```python
from build123d import *

# Parameters (mm, degrees)
BOSS_EXTRUDE1_DEPTH = 50.8
SKETCH4_R           = 2.667
CUT_EXTRUDE1_DEPTH  = 117.743329574
SKETCH5_W           = 88.9
SKETCH5_H           = 38.1
CUT_EXTRUDE2_DEPTH  = 20.32
SKETCH6_W           = 88.9
SKETCH6_H           = 38.1
CUT_EXTRUDE3_DEPTH  = 20.32
SKETCH7_R           = 3.175
CUT_EXTRUDE4_DEPTH  = 117.743329574


with BuildPart() as part:
    # Sketch3 → Boss-Extrude1 (new body)
    with BuildSketch(Plane.XY):
        Polygon((0, 6.35), (88.9, 44.45), (95.25, 44.45), (95.25, 0), (0, 0), align=None)
        Polygon((16.120053074, 6.35), (88.9, 6.35), (88.9, 37.541405825), align=None, mode=Mode.SUBTRACT)
    extrude(amount=BOSS_EXTRUDE1_DEPTH)

    # Sketch4 → Cut-Extrude1 (cut, through all)
    with BuildSketch(Plane.XZ):
        with Locations(Location((6.35, 38.1, 0), (0, 0, 270))):
            Circle(SKETCH4_R)
        with Locations(Location((6.35, 12.7, 0), (0, 0, 270))):
            Circle(SKETCH4_R)
        with Locations(Location((69.85, 12.7, 0), (0, 0, 270))):
            Circle(SKETCH4_R)
        with Locations(Location((69.85, 38.1, 0), (0, 0, 270))):
            Circle(SKETCH4_R)
    extrude(amount=-CUT_EXTRUDE1_DEPTH, mode=Mode.SUBTRACT)

    # Sketch5 → Cut-Extrude2 (cut)
    with BuildSketch(Plane.XY.offset(50.8)):
        with Locations((44.45, 25.4)):
            Rectangle(SKETCH5_W, SKETCH5_H)
    extrude(amount=-CUT_EXTRUDE2_DEPTH, mode=Mode.SUBTRACT)

    # Sketch6 → Cut-Extrude3 (cut)
    with BuildSketch(Plane(origin=(0, 0, 0), x_dir=(-1, 0, 0), z_dir=(0, 0, -1))):
        with Locations((-44.45, 25.4)):
            Rectangle(SKETCH6_W, SKETCH6_H)
    extrude(amount=-CUT_EXTRUDE3_DEPTH, mode=Mode.SUBTRACT)

    # Sketch7 → Cut-Extrude4 (cut, through all)
    with BuildSketch(Plane(origin=(95.25, 0, 0), x_dir=(0, 0, -1), z_dir=(1, 0, 0))):
        with Locations((-38.1, 15.24)):
            Circle(SKETCH7_R)
        with Locations((-12.7, 15.24)):
            Circle(SKETCH7_R)
        with Locations((-12.7, 34.29)):
            Circle(SKETCH7_R)
        with Locations((-38.1, 34.29)):
            Circle(SKETCH7_R)
    extrude(amount=-CUT_EXTRUDE4_DEPTH, mode=Mode.SUBTRACT)


solid = part.part
```
Verification items for the finished model (mm, model axes). A direction names the side the tool comes from. Give positions to 0.01 mm unless a question says otherwise; leave off trailing zeros. Loops run counter-clockwise (first coordinate to the right, second up) from the corner with the lowest first, then second, coordinate; pieces in that order, holes last. Notation, with made-up numbers: M 82.5,37 L 137.5,37 A25 cw 137.5,58 Z; hole C -12,-9 d3. An arc over 180 degrees is marked long. Return JSON: item names as keys, results as strings.
1) Section check A-A, the plane z = 12.7. Enter the section's corners in (x, y) (3 decimals), and give its area (3 significant figures).
Findings:
{"outline": "M 0,0 L 3.683,0 L 3.683,6.35 L 0,6.35 Z; M 9.017,0 L 67.183,0 L 67.183,6.35 L 9.017,6.35 Z; M 72.517,0 L 95.25,0 L 95.25,12.065 L 88.9,12.065 L 88.9,6.35 L 72.517,6.35 Z; M 88.9,18.415 L 95.25,18.415 L 95.25,31.115 L 88.9,31.115 Z; M 88.9,37.465 L 95.25,37.465 L 95.25,44.45 L 88.9,44.45 Z", "area": "698 mm2"}
2) Section check B-B, the plane x = 6.35. Enter the section's corners in (y, z).
Findings:
{"outline": "M 0,0 L 6.35,0 L 6.35,10.03 L 0,10.03 Z; M 0,15.37 L 6.35,15.37 L 6.35,20.32 L 9.07,20.32 L 9.07,30.48 L 6.35,30.48 L 6.35,35.43 L 0,35.43 Z; M 0,40.77 L 6.35,40.77 L 6.35,50.8 L 0,50.8 Z"}
3) Section check D-D, the plane z = 28. Enter the section's corners in (x, y).
Findings:
{"outline": "M 0,0 L 95.25,0 L 95.25,44.45 L 88.9,44.45 L 0,6.35 Z; hole M 16.12,6.35 L 88.9,6.35 L 88.9,37.54 Z"}
4) Section check C-C, the plane y = 9. Enter the section's corners in (x, z), and give its area (3 significant figures).
Findings:
{"outline": "M 6.18,20.32 L 22.3,20.32 L 22.3,30.48 L 6.18,30.48 Z; M 88.9,0 L 95.25,0 L 95.25,50.8 L 88.9,50.8 Z", "area": "486 mm2"}
5) Material ranges on L1, parallel to X at y = 4.5, z = 12.7; L2, parallel to Y at x = 90.75, z = 38.1 (3 decimals); L3, parallel to Z at x = 6, y = 4, recorded low to high. Write a range as [from, to].
Findings:
{"L1": "x = [0, 3.68], [9.02, 67.18], [72.52, 95.25]", "L2": "y = [0, 12.065], [18.415, 31.115], [37.465, 44.45]", "L3": "z = [0, 10.06], [15.34, 35.46], [40.74, 50.8]"}
6) Gauge pin test, flat ends, axial feed: P1, Ø8.5, axis at x = 69.85, z = 12.7, coming from the +Y side; P2, Ø8.5, axis at y = 34.29, z = 12.7, coming from the -X side; P3, Ø19, axis at y = 25.5, z = 26, coming from the -X side. Record the tip position at first contact, or that the pin passes through.
Findings:
{"P1": "stops at y = 6.35", "P2": "stops at x = 88.9", "P3": "stops at x = 22.52"}
7) Mould release check, pull along Y, two halves, no side actions. Record for faces 4 (the cylindrical face through (92.12, 12.14, 13.39)), 5 (the flat face through (92, 44.45, 25)), 6 (the flat face through (95.25, 23, 25)): released by +Y, released by -Y, zero draft, split by the parting line, or undercut.
Findings:
{"face 4": "undercut", "face 5": "released by +Y", "face 6": "zero draft"}
8) Tool access check on faces 1 (the flat face through (48, 24, 20.32)), 2 (the flat face through (53.019, 22.164, 25.329)), 3 (the flat face through (48, 23, 30.48)). Record the directions out of +Z, -Z, +X, -X, +Y, -Y that give a thin tool (end or side, any length) a straight path to the whole face; none if there is none.
Findings:
{"face 1": "-Z, -X, +Y", "face 2": "+Z, -Z", "face 3": "+Z, -X, +Y"}
